from build123d import *

# Parameters (mm, degrees)
EXTRUDE_1_DEPTH = 7
SKETCH_2_R      = 9
EXTRUDE_2_DEPTH = 7
SKETCH_3_R      = 7.2
EXTRUDE_3_DEPTH = 26
SKETCH_4_R      = 3.7
EXTRUDE_4_DEPTH = 3


with BuildPart() as part:
    # 草图1 → 凸台-拉伸1 (new body)
    with BuildSketch(Plane(origin=(0, 0, 0), x_dir=(1, 0, 0), z_dir=(0, 1, 0))):
        Polygon((6.325906751, 8.245174576), (-3.977577266, 9.600983236), (-10.303484016, 1.35580866), (-6.325906751, -8.245174576), (3.977577266, -9.600983236), (10.303484016, -1.35580866), align=None)
    extrude(amount=EXTRUDE_1_DEPTH)

    # 草图2 → 凸台-拉伸2 (add)
    with BuildSketch(Plane.XZ):
        with Locations(Location((0, 0, 0), (0, 0, 97.49633363))):
            Circle(SKETCH_2_R)
    extrude(amount=EXTRUDE_2_DEPTH)

    # 草图3 → 凸台-拉伸3 (add)
    with BuildSketch(Plane.XZ.offset(7)):
        with Locations(Location((0, 0, 0), (0, 0, 90))):
            Circle(SKETCH_3_R)
    extrude(amount=EXTRUDE_3_DEPTH)

    # 草图4 → 凸台-拉伸4 (add)
    with BuildSketch(Plane.XZ.offset(33)):
        with Locations(Location((0, 0, 0), (0, 0, 270))):
            Circle(SKETCH_4_R)
    extrude(amount=EXTRUDE_4_DEPTH)


solid = part.part
Model file for the job. Use its own axes, mm. A direction names the side the tool comes from. Round coordinates to 2 decimals unless told otherwise and drop trailing zeros. Order: outer loops, then holes, each group sorted by start corner. A loop starts at its lowest first (then second) coordinate and runs counter-clockwise, first axis right, second up.
(1) 3-axis set-ups, long thin cutter, end or side, ignore diameter. For faces 1 (the face through (6, 0, -7)), 2 (the face through (-6, 0, 7)), 3 (the face through (3, -33, 3)): which of +Z, -Z, +X, -X, +Y, -Y reach the whole face in a straight line?
(2) Pin check, flat tips, straight feed: pin 1 (4 mm diameter, centred on y = -21, z = 0.5, fed in from +X); pin 2 (8 mm diameter, centred on y = -31.5, z = 5.5, fed in from +X); pin 3 (1.6 mm diameter, centred on x = 3, z = -7, fed in from -Y). Stop position of each tip, or through.
(3) Band-saw the part on D-D (z = 0). List the corners of the cut face in (x, y).
(4) Drill centre lines: line 1 (Y direction, x = 6.75, z = 1.25); line 2 (Y direction, x = -4.5, z = -7.75); line 3 (Z direction, x = -6, y = -25). Where is each one in solid material? Low to high.
(5) Band-saw the part on C-C (y = -12.5). List the corners of the cut face in (x, z).
(6) Band-saw the part on A-A (z = 6.5). List the corners of the cut face in (x, y).
(7) Band-saw the part on B-B (x = 0). List the corners of the cut face in (y, z), then the cut area to 3 significant figures.
Verdict:
1. face 1: -Z, +X, -Y
1. face 2: +Z, -X, -Y
1. face 3: -Y
2. pin 1: stops at x = 7.2
2. pin 2: stops at x = 7.04
2. pin 3: stops at y = -33
3. outline: (-9.74, 0) - (-9, 0) - (-9, -7) - (-7.2, -7) - (-7.2, -33) - (-3.7, -33) - (-3.7, -36) - (3.7, -36) - (3.7, -33) - (7.2, -33) - (7.2, -7) - (9, -7) - (9, 0) - (9.74, 0) - (9.74, 7) - (-9.74, 7) - close
4. line 1: y = -33 to 7
4. line 2: y = -7 to 7
4. line 3: z = -3.98 to 3.98
5. outline: circle Ø14.4 at (0, 0)
6. outline: (-7.05, 0) - (-6.22, 0) - (-6.22, -7) - (-3.1, -7) - (-3.1, -33) - (3.1, -33) - (3.1, -7) - (6.22, -7) - (6.22, 0) - (6.36, 0) - (6.36, 7) - (-7.05, 7) - close
7. outline: (-36, -3.7) - (-33, -3.7) - (-33, -7.2) - (-7, -7.2) - (-7, -9) - (0, -9) - (0, -9.08) - (7, -9.08) - (7, 9.08) - (0, 9.08) - (0, 9) - (-7, 9) - (-7, 7.2) - (-33, 7.2) - (-33, 3.7) - (-36, 3.7) - close
7. area: 650 mm2
